Geometry: final body of the model. Coordinates: model frame, mm. Face numbers are marked on the shaded views. Coordinates: 2 decimals unless noted, no trailing zeros. Loops run counter-clockwise (first coordinate to the right, second up) from the corner with the lowest first, then second, coordinate; pieces in that order, holes last. Notation, with made-up numbers: (-13.75, -30.5) -> (43.25, -30.5) arc R27 ccw to (43.25, -14.5) -> close; hole circle Ø2 at (44.5, 46.5). An arc over 180 degrees is marked (long way). One line per item, written item: value. Start each with the question number.
Item 1: Ray query, probe 1 along Y at (x, z) = (0, 0.9); probe 2 along X at (y, z) = (-2.5, 1.35); probe 3 along Y at (x, z) = (2, 1.1). Return the intervals inside material, ascending. Write a range as from..to.
Item 2: Contact query for a flat-ended pin moving along its axis: pin 1 Ø1 at (y, z) = (1, 1) entering from +X. Output: stop coordinate, or through.
Item 3: Section query D-D on z = 1.7. Return loops of the section in (x, y), then the cut area to 3 significant figures.
Item 4: Section query C-C on z = 0.8. Return loops of the section in (x, y).
Item 5: Section query A-A on y = 0. Return loops of the section in (x, z).
Item 6: Mould query, pull axis X, two halves, no side actions, for the marked faces 1, 2 and 3. Classes: +X half, -X half, draft (parallel to the pull), parting line (faces both ways), or undercut.
from build123d import *

# Parameters (mm, degrees)
SKETCH1_R           = 4.25
SKETCH1_R_2         = 3
BOSS_EXTRUDE2_DEPTH = 2
FILLET3_R           = 1
FILLET4_R           = 0.5


with BuildPart() as part:
    # Sketch1 → Boss-Extrude2 (new body)
    with BuildSketch(Plane.XY):
        Circle(SKETCH1_R)
        Circle(SKETCH1_R_2, mode=Mode.SUBTRACT)
    extrude(amount=BOSS_EXTRUDE2_DEPTH)

    # Fillet3
    fillet3_edges = [part.edges().sort_by_distance(p)[0] for p in [
        (-4.25, 0, 2),
    ]]
    fillet(fillet3_edges, radius=FILLET3_R)

    # Fillet4
    fillet4_edges = [part.edges().sort_by_distance(p)[0] for p in [
        (-4.25, 0, 0),
    ]]
    fillet(fillet4_edges, radius=FILLET4_R)


solid = part.part
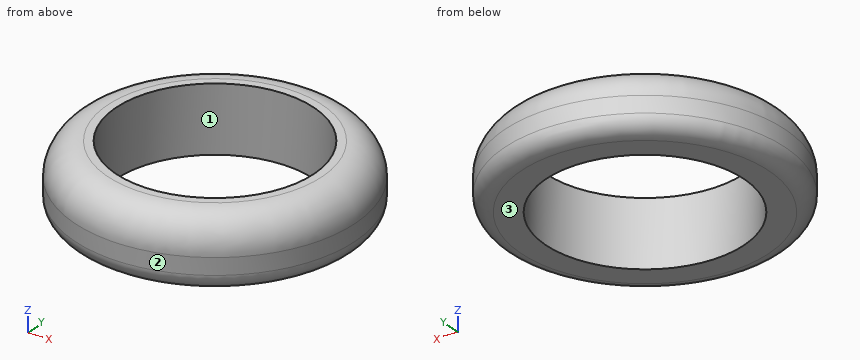
Reply:
1. probe 1: y = -4.25..-3, 3..4.25
1. probe 2: x = -3.36..-1.66, 1.66..3.36
1. probe 3: y = -3.74..-2.24, 2.24..3.74
2. pin 1: stops at x = 4.22
3. outline: circle Ø7.93 at (0, 0); hole circle Ø6 at (0, 0)
3. area: 21.1 mm²
4. outline: circle Ø8.5 at (0, 0); hole circle Ø6 at (0, 0)
5. outline: (-4.25, 0.5) arc R0.5 ccw to (-3.75, 0) -> (-3, 0) -> (-3, 2) -> (-3.25, 2) arc R1 ccw to (-4.25, 1) -> close; (3, 0) -> (3.75, 0) arc R0.5 ccw to (4.25, 0.5) -> (4.25, 1) arc R1 ccw to (3.25, 2) -> (3, 2) -> close
6. face 1: undercut
6. face 2: parting line
6. face 3: draft
